Build history of the part. All positions in model axes, mm. Face numbers are marked on the shaded views. A direction names the side the tool comes from. Round coordinates to 2 decimals unless told otherwise and drop trailing zeros. Write each loop counter-clockwise with the first axis right and the second up, starting at its lowest first coordinate (ties: lowest second). Pieces come first, ordered by that corner, then holes. Notation, with made-up numbers: M -27,30 L -18,30 A4 ccw -18,35 Z; hole C -26,85.5 d1. An arc over 180 degrees is marked long. Write item = value, one per line. Start each with the question number.
Q1. Band-saw the part on B-B on x = 5. Write the cut outline in (y, z).
Q2. Band-saw the part on D-D on x = 3. Write the cut outline in (y, z).
Q3. Pull direction X, two halves, no side cores. Call the marked faces 4, 5 and 6: released by +X, released by -X, zero draft, split by the parting line, or undercut.
Q4. Band-saw the part on C-C on y = 4. Write the cut outline in (x, z).
Q5. Drop flat-ended pins along their axis: P1, Ø1.6, axis at x = 3, z = -3.5, coming from the +Y side; P2, Ø1, axis at x = 7.5, y = 2.5, coming from the +Z side; P3, Ø0.5, axis at x = 6.5, z = -0.5, coming from the -Y side. Give the stop position or say it passes through.
Q6. Tool access for the marked faces 1, 2 and 3: list every direction of +Z, -Z, +X, -X, +Y, -Y with a clear straight run to the whole face (end or side of a thin tool).
Q7. Probe L1, parallel to X at y = 8.9, z = -3.5; L2, parallel to Z at x = 4.25, y = 2.5; L3, parallel to Y at x = 7.25, z = -3.75. List the from-to ranges inside material, lowest first.
Q8. Band-saw the part on A-A on z = -3.5. Write the cut outline in (x, y), plus the area to 3 significant figures.
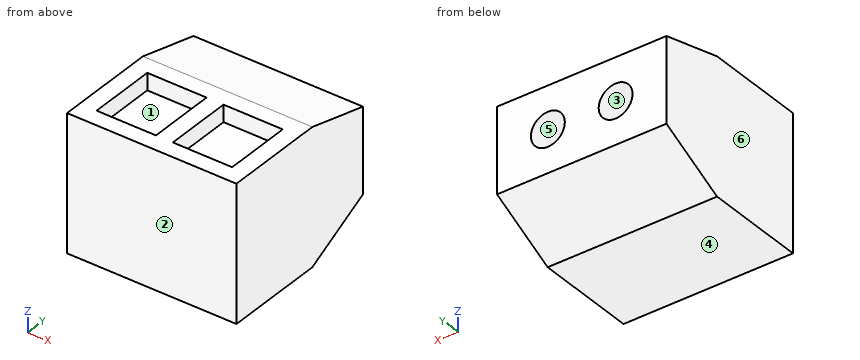
```python
from build123d import *

# Parameters (mm, degrees)
SKETCH1_W           = 10
SKETCH1_H           = 8
BOSS_EXTRUDE1_DEPTH = 10
CUT_EXTRUDE1_DEPTH  = 10
SKETCH4_R           = 1
CUT_EXTRUDE2_DEPTH  = 2
SKETCH5_W           = 3.5
SKETCH5_H           = 4
CUT_EXTRUDE3_DEPTH  = 1


with BuildPart() as part:
    # Sketch1 → Boss-Extrude1 (new body)
    with BuildSketch(Plane(origin=(0, 0, 0), x_dir=(1, 0, 0), z_dir=(0, 1, 0))):
        with Locations((5, 4)):
            Rectangle(SKETCH1_W, SKETCH1_H)
    extrude(amount=BOSS_EXTRUDE1_DEPTH)

    # Sketch3 → Cut-Extrude1 (cut)
    with BuildSketch(Plane(origin=(10, 0, 0), x_dir=(0, 0, -1), z_dir=(1, 0, 0))):
        Polygon((0, 6), (1, 10), (6, 10), (8, 6), (9, 6), (9, 11), (-1, 11), (-1, 6), align=None)
    extrude(amount=-CUT_EXTRUDE1_DEPTH, mode=Mode.SUBTRACT)

    # Sketch4 → Cut-Extrude2 (cut)
    with BuildSketch(Plane(origin=(0, 10, 0), x_dir=(1, 0, 0), z_dir=(0, 1, 0))):
        with Locations(Location((3, 3.5, 0), (0, 0, 270))):
            Circle(SKETCH4_R)
        with Locations(Location((7, 3.5, 0), (0, 0, 270))):
            Circle(SKETCH4_R)
    extrude(amount=-CUT_EXTRUDE2_DEPTH, mode=Mode.SUBTRACT)

    # Sketch5 → Cut-Extrude3 (cut)
    with BuildSketch(Plane.XY):
        with Locations((2.75, 3)):
            Rectangle(SKETCH5_W, SKETCH5_H)
        with Locations((7.25, 3)):
            Rectangle(SKETCH5_W, SKETCH5_H)
    extrude(amount=-CUT_EXTRUDE3_DEPTH, mode=Mode.SUBTRACT)


solid = part.part
```
Conclusion:
q1.outline = M 0,-8 L 6,-8 L 10,-6 L 10,-1 L 6,0 L 0,0 Z
q2.outline = M 0,-8 L 6,-8 L 10,-6 L 10,-4.5 L 8,-4.5 L 8,-2.5 L 10,-2.5 L 10,-1 L 6,0 L 5,0 L 5,-1 L 1,-1 L 1,0 L 0,0 Z
q3.face_4 = zero draft
q3.face_5 = undercut
q3.face_6 = released by -X
q4.outline = M 0,-8 L 10,-8 L 10,0 L 9,0 L 9,-1 L 5.5,-1 L 5.5,0 L 4.5,0 L 4.5,-1 L 1,-1 L 1,0 L 0,0 Z
q5.P1 = 8
q5.P2 = -1
q5.P3 = 0
q6.face_1 = +Z
q6.face_2 = +Z, -Z, +X, -X, -Y
q6.face_3 = +Y
q7.L1 = 0 to 2, 4 to 6, 8 to 10
q7.L2 = -8 to -1
q7.L3 = 0 to 8
q8.outline = M 0,0 L 10,0 L 10,10 L 8,10 L 8,8 L 6,8 L 6,10 L 4,10 L 4,8 L 2,8 L 2,10 L 0,10 Z
q8.area = 92.0 mm^2
